The drawing under review shows one solid part. Ordinate dimensions are in mm from its lowest x, y, z. A direction names the side the tool comes from. Round coordinates to 2 decimals unless told otherwise and drop trailing zeros. Write each loop counter-clockwise with the first axis right and the second up, starting at its lowest first coordinate (ties: lowest second). Pieces come first, ordered by that corner, then holes. Notation, with made-up numbers: (6, 58.5) - (25, 58.5) arc R32 ccw to (25, 95.5) - close; hole circle Ø1 at (14.25, 46). An arc over 180 degrees is marked (long way). One line per question, with ' | ' between items. Start each with the question number.
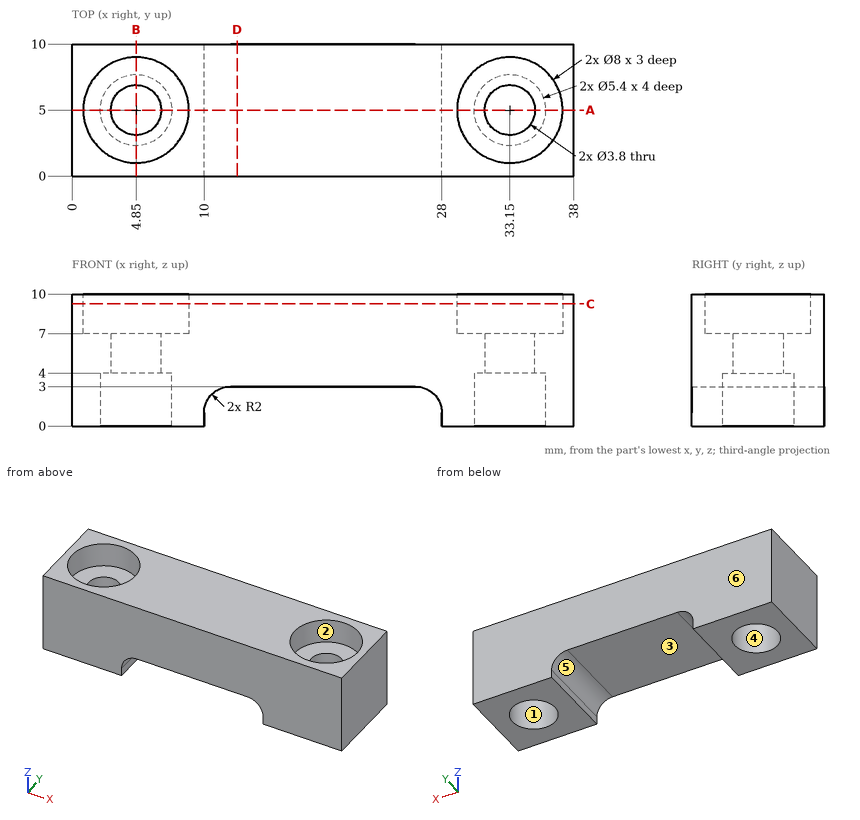
1. The part is to be moulded in two halves that separate along Y. For the marked faces 4, 5 and 6, say which applies: pulls with the +Y half, pulls with the -Y half, needs draft (parallel to the pull), parting line crosses it, or undercut.
2. Add section A-A, the plane y = 5. State how many separate pieces and enclosed holes the cut face has, then the cut area to 3 significant figures.
3. Add section C-C, the plane z = 9.25. Write out the cut boundary in (x, y).
4. Add section D-D, the plane x = 12.5. Write out the cut boundary in (y, z).
5. Clearance check with a flat-ended pin moving along its axis: P1, Ø2.5, axis at x = 4, y = 5, coming from the -Z side. State where the tip first meets the part, or that it passes through.
6. Machinability: for the marked faces 1, 2 and 3, which of the approach directions +Z, -Z, +X, -X, +Y, -Y give a long, thin tool a straight path to every point of the face, cutting with its end or side? Answer none if there is none.
7. Wall thickness on line 1 along X through (y, z) = (5, 5.4); line 2 along X through (y, z) = (1.5, 8.5); line 3 along X through (y, z) = (7, 2.75): over which ranges is each line inside the solid? List them lowest first. Write a range as [from, to].
8. Add section B-B, the plane x = 4.85. Write out the cut boundary in (y, z).
Geometry check:
1) face 4: undercut | face 5: needs draft | face 6: pulls with the +Y half
2) separate pieces: 3 | enclosed holes: 0 | area: 214 mm2
3) outline: (0, 0) - (38, 0) - (38, 10) - (0, 10) - close; hole circle Ø8 at (4.85, 5); hole circle Ø8 at (33.15, 5)
4) outline: (0, 3) - (10, 3) - (10, 10) - (0, 10) - close
5) P1: stops at z = 4
6) face 1: -Z | face 2: +Z | face 3: -Z, +Y, -Y
7) line 1: x = [0, 2.95], [6.75, 31.25], [35.05, 38] | line 2: x = [0, 2.91], [6.79, 31.21], [35.09, 38] | line 3: x = [0, 3.04], [6.66, 11.03], [26.97, 31.34], [34.96, 38]
8) outline: (0, 0) - (2.3, 0) - (2.3, 4) - (3.1, 4) - (3.1, 7) - (1, 7) - (1, 10) - (0, 10) - close; (6.9, 4) - (7.7, 4) - (7.7, 0) - (10, 0) - (10, 10) - (9, 10) - (9, 7) - (6.9, 7) - close
